Model file for the job. Use its own axes, mm. A direction names the side the tool comes from. Give positions to 0.01 mm unless a question says otherwise; leave off trailing zeros. Write each loop counter-clockwise with the first axis right and the second up, starting at its lowest first coordinate (ties: lowest second). Pieces come first, ordered by that corner, then holes.
```python
from build123d import *

# Parameters (mm, degrees)
F0_W     = 10
F0_H     = 36
F1_DEPTH = 4
F2_R     = 1
F3_R     = 1
F4_R     = 1.5


with BuildPart() as f1:
    # F0 (on Front) → F1 (new body)
    with BuildSketch(Plane.XZ):
        with BuildLine():
            ThreePointArc((-18.134615, -17.951065), (-16.670149, -21.486599), (-13.134615, -22.951065))
            Line((-13.134615, -22.951065), (16.865385, -22.951065))
            ThreePointArc((16.865385, -22.951065), (20.400919, -21.486599), (21.865385, -17.951065))
            Line((21.865385, -17.951065), (21.865385, 17.048935))
            ThreePointArc((21.865385, 17.048935), (20.400919, 20.584469), (16.865385, 22.048935))
            Line((16.865385, 22.048935), (-13.134615, 22.048935))
            ThreePointArc((-13.134615, 22.048935), (-16.670149, 20.584469), (-18.134615, 17.048935))
            Line((-18.134615, 17.048935), (-18.134615, -17.951065))
        make_face()
        with Locations((-5.634615, -0.451065)):
            Rectangle(F0_W, F0_H, mode=Mode.SUBTRACT)
        with Locations((9.365385, -0.451065)):
            Rectangle(F0_W, F0_H, mode=Mode.SUBTRACT)
    extrude(amount=F1_DEPTH)

    # F2
    f2_edges = [f1.edges().sort_by_distance(p)[0] for p in [
        (-0.634615, 0, -0.451065),
        (4.365385, 0, -0.451065),
        (4.365385, -4, -0.451065),
        (-0.634615, -4, -0.451065),
    ]]
    fillet(f2_edges, radius=F2_R)

    # F3
    f3_edges = [f1.edges().sort_by_distance(p)[0] for p in [
        (14.365385, -4, -0.451065),
        (14.365385, 0, -0.451065),
        (-10.634615, -4, -0.451065),
        (-10.634615, 0, -0.451065),
    ]]
    fillet(f3_edges, radius=F3_R)

    # F4
    f4_edges = [f1.edges().sort_by_distance(p)[0] for p in [
        (21.865385, -4, -0.451065),
        (21.865385, 0, -0.451065),
    ]]
    fillet(f4_edges, radius=F4_R)


solid = f1.part
```
1. Probe probe 1 along X at (y, z) = (-2.6, -15.5); probe 2 along X at (y, z) = (-3.55, 10.5); probe 3 along Z at (x, y) = (-8, -1.5). List the from-to ranges inside material, lowest first.
Calculated:
probe 1: x = -18.13 to -10.63, -0.63 to 4.37, 14.37 to 21.86
probe 2: x = -17.71 to -10.8, -0.47 to 4.2, 14.53 to 21.44
probe 3: z = -22.95 to -18.45, 17.55 to 22.05
2. Slice it at A-A, the plane z = 12.5. Write the cut outline in (x, y), and give its area (3 significant figures).
Calculated:
outline: (-18.13, -2.5) arc R1.5 ccw to (-16.63, -4) - (-11.63, -4) arc R1 ccw to (-10.63, -3) - (-10.63, -1) arc R1 ccw to (-11.63, 0) - (-16.63, 0) arc R1.5 ccw to (-18.13, -1.5) - close; (-0.63, -3) arc R1 ccw to (0.37, -4) - (3.37, -4) arc R1 ccw to (4.37, -3) - (4.37, -1) arc R1 ccw to (3.37, 0) - (0.37, 0) arc R1 ccw to (-0.63, -1) - close; (14.37, -3) arc R1 ccw to (15.37, -4) - (20.37, -4) arc R1.5 ccw to (21.87, -2.5) - (21.87, -1.5) arc R1.5 ccw to (20.37, 0) - (15.37, 0) arc R1 ccw to (14.37, -1) - close
area: 76.4 mm2
3. Pin check, flat tip, straight feed: P1, Ø3, axis at x = -9.5, z = -6, coming from the +Y side. Stop position of the tip, or through.
Calculated:
P1: stops at y = -0.23
4. Pull direction X, two halves, no side cores. Call faces 5 (the flat face through (9, -2, 17.549)), 6 (the flat face through (-18.135, -2, 0)), 7 (the flat face through (2, -2, 22.049)), 8 (the cylindrical face through (21.414, -0.428, -0.206)): +X half, -X half, draft (parallel to the pull), parting line (faces both ways), or undercut.
Calculated:
face 5: undercut
face 6: -X half
face 7: draft
face 8: +X half
5. Which spindle directions (+Z, -Z, +X, -X, +Y, -Y) get a long thin tool onto all of the face, cutting with end or side? Do faces 1 (the cylindrical face through (4.08, -0.3, -0.2)), 2 (the cylindrical face through (4.08, -3.7, -0.2)), 3 (the flat face through (2, 0, 0)), 4 (the flat face through (-10.635, -2, -1)). Say none if no direction does.
Calculated:
face 1: +Y
face 2: -Y
face 3: +Z, -Z, +X, -X, +Y
face 4: +Y, -Y
6. Slice it at B-B, the plane x = -5.5. Write the cut outline in (y, z), and give its area (3 significant figures).
Calculated:
outline: (-4, -21.45) arc R1.5 ccw to (-2.5, -22.95) - (-1.5, -22.95) arc R1.5 ccw to (0, -21.45) - (0, -18.45) - (-4, -18.45) - close; (-4, 17.55) - (0, 17.55) - (0, 20.55) arc R1.5 ccw to (-1.5, 22.05) - (-2.5, 22.05) arc R1.5 ccw to (-4, 20.55) - close
area: 34.1 mm2
